Model file for the job. Use its own axes, mm. Face numbers are marked on the shaded views. A direction names the side the tool comes from. Give positions to 0.01 mm unless a question says otherwise; leave off trailing zeros. Order: outer loops, then holes, each group sorted by start corner. A loop starts at its lowest first (then second) coordinate and runs counter-clockwise, first axis right, second up. Notation, with made-up numbers: M -24,11 L 27,11 A28 cw 27,36 Z; hole C -8,-8.75 d6. An arc over 180 degrees is marked long. Return JSON: item names as keys, results as strings. Group by question number.
1. Pin check, flat tips, straight feed: pin 1 (10 mm diameter, centred on x = 34.5, y = -119.5, fed in from -Z); pin 2 (10 mm diameter, centred on x = -18, y = -134.5, fed in from +Z) (3 decimals); pin 3 (10.5 mm diameter, centred on y = -44.5, z = 24.5, fed in from -X) (3 decimals); pin 4 (2.5 mm diameter, centred on x = -32, z = 1, fed in from +Y). Stop position of each tip, or through.
2. 3-axis set-ups, long thin cutter, end or side, ignore diameter. For the marked faces 4 and 5: which of +Z, -Z, +X, -X, +Y, -Y reach the whole face in a straight line?
3. Slice it at C-C on x = -28.5. List the corners of the cut face in (y, z) (3 decimals).
4. Slice it at B-B on z = 5.5. List the corners of the cut face in (x, y) (3 decimals), then the cut area to 3 significant figures.
5. Two-plate mould, pull along X, no slides. Class the marked faces 1, 2 and 3: released by +X, released by -X, zero draft, split by the parting line, or undercut.
6. Wall check: probe 1 along X at (y, z) = (-105, 16) (3 decimals); probe 2 along X at (y, z) = (-66, 17) (3 decimals); probe 3 along Z at (x, y) = (5, -37) (3 decimals). Give the ranges that are in metal, low to high. Write a range as [from, to].
7. Slice it at D-D on z = 25.5. List the corners of the cut face in (x, y) (3 decimals).
8. Slice it at A-A on y = -54.5. List the corners of the cut face in (x, z) (3 decimals), then the cut area to 3 significant figures.
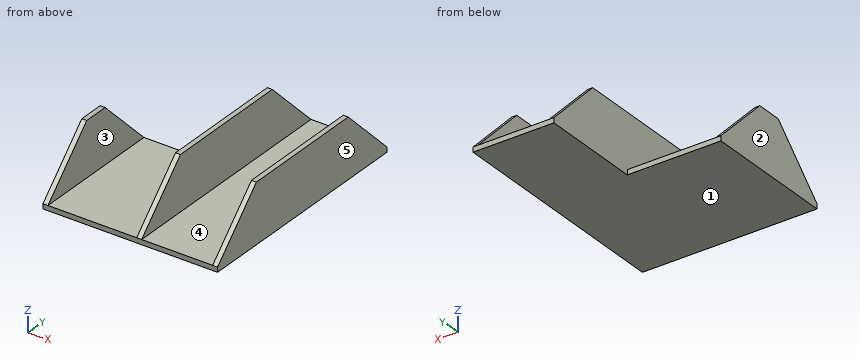
from build123d import *

# Parameters (mm, degrees)
F0_W     = 45.72
F0_H     = 152.4
F1_DEPTH = 3.175
F3_DEPTH = 3.175
F5_DEPTH = 3.175
F6_W     = 57.15
F6_H     = 86.36
F7_DEPTH = 3.175
F9_DEPTH = 3.175


with BuildPart() as f1:
    # F0 (on Top) → F1 (new body)
    with BuildSketch(Plane.XY):
        with Locations((22.86, -76.2)):
            Rectangle(F0_W, F0_H)
    extrude(amount=F1_DEPTH)

    # F2 (on face) → F3 (join)
    with BuildSketch(Plane.YZ.offset(45.72)):
        Polygon((-152.4, 3.175), (-152.4, 0), (0, 0), (0, 3.175), (-34.925, 38.1), (-117.475, 38.1), align=None)
    extrude(amount=F3_DEPTH)

    # F4 (on face) → F5 (join)
    with BuildSketch(Plane(origin=(0, 0, 0), x_dir=(0, -1, 0), z_dir=(-1, 0, 0))):
        Polygon((34.925, 38.1), (0, 3.175), (152.4, 3.175), (117.475, 38.1), align=None)
        Polygon((0, 3.175), (0, 0), (152.4, 0), (152.4, 3.175), (117.475, 38.1), (34.925, 38.1), align=None)
    extrude(amount=F5_DEPTH)

    # F6 (on face) → F7 (join)
    with BuildSketch(Plane(origin=(0, 0, 0), x_dir=(1, 0, 0), z_dir=(0, 0, -1))):
        with Locations((-31.75, 109.22)):
            Rectangle(F6_W, F6_H)
    extrude(amount=-F7_DEPTH)

    # F8 (on face) → F9 (join)
    with BuildSketch(Plane(origin=(-60.325, 0, 0), x_dir=(0, -1, 0), z_dir=(-1, 0, 0))):
        Polygon((66.04, 0), (152.4, 0), (152.4, 3.175), (117.475, 38.1), (100.965, 38.1), (66.04, 3.175), align=None)
    extrude(amount=F9_DEPTH)


solid = f1.part
Result:
{
 "1": {"pin 1": "stops at z = 0", "pin 2": "stops at z = 3.175", "pin 3": "stops at x = -3.175", "pin 4": "stops at y = -66.04"},
 "2": {"face 4": "+Z, +Y, -Y", "face 5": "+Z, -Z, +X, +Y, -Y"},
 "3": {"outline": "M -152.4,0 L -66.04,0 L -66.04,3.175 L -152.4,3.175 Z"},
 "4": {"outline": "M -63.5,-150.075 L -60.325,-150.075 L -60.325,-68.365 L -63.5,-68.365 Z; M -3.175,-150.075 L 0,-150.075 L 0,-2.325 L -3.175,-2.325 Z; M 45.72,-150.075 L 48.895,-150.075 L 48.895,-2.325 L 45.72,-2.325 Z", "area": "1,200 mm2"},
 "5": {"face 1": "zero draft", "face 2": "released by -X", "face 3": "undercut"},
 "6": {"probe 1": "x = [-63.5, -60.325], [-3.175, 0], [45.72, 48.895]", "probe 2": "x = [-3.175, 0], [45.72, 48.895]", "probe 3": "z = [0, 3.175]"},
 "7": {"outline": "M -63.5,-130.075 L -60.325,-130.075 L -60.325,-88.365 L -63.5,-88.365 Z; M -3.175,-130.075 L 0,-130.075 L 0,-22.325 L -3.175,-22.325 Z; M 45.72,-130.075 L 48.895,-130.075 L 48.895,-22.325 L 45.72,-22.325 Z"},
 "8": {"outline": "M -3.175,0 L 48.895,0 L 48.895,38.1 L 45.72,38.1 L 45.72,3.175 L 0,3.175 L 0,38.1 L -3.175,38.1 Z", "area": "387 mm2"}
}
